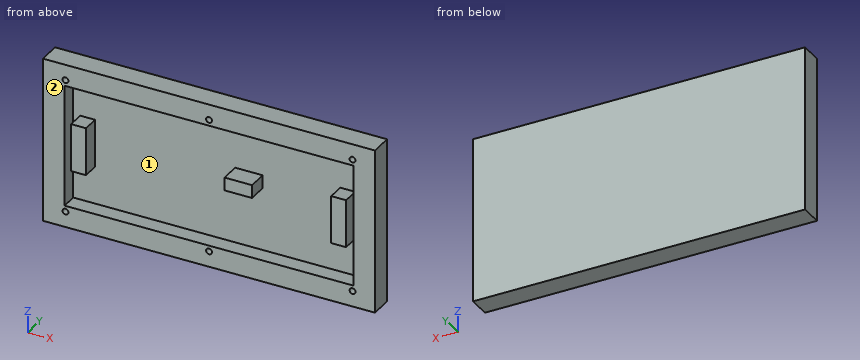
```python
from build123d import *

# Parameters (mm, degrees)
SKETCH1_W                = 192
SKETCH1_H                = 96
BOSS_EXTRUDE1_DEPTH      = 12.8
SKETCH2_W                = 167
SKETCH2_H                = 71
CUT_EXTRUDE1_DEPTH       = 9.2
M3_CLEARANCE_HOLE1_D     = 3.4
M3_CLEARANCE_HOLE1_DEPTH = 5
M3_CLEARANCE_HOLE1_TIP   = 1.021463052
SKETCH6_W                = 8.6
SKETCH6_H                = 27.8
BOSS_EXTRUDE2_DEPTH      = 9.6
SKETCH7_W                = 15.9
SKETCH7_H                = 7.6
BOSS_EXTRUDE3_DEPTH      = 11.2


with BuildPart() as part:
    # Sketch1 → Boss-Extrude1 (new body)
    with BuildSketch(Plane(origin=(0, 0, 0), x_dir=(1, 0, 0), z_dir=(0, 1, 0))):
        with Locations((96, 48)):
            Rectangle(SKETCH1_W, SKETCH1_H)
    extrude(amount=BOSS_EXTRUDE1_DEPTH)

    # Sketch2 → Cut-Extrude1 (cut)
    with BuildSketch(Plane.XZ):
        with Locations((96, -48)):
            Rectangle(SKETCH2_W, SKETCH2_H)
    extrude(amount=-CUT_EXTRUDE1_DEPTH, mode=Mode.SUBTRACT)

    # M3 Clearance Hole1
    with Locations(Plane(origin=(0, 0, 0), x_dir=(-1, 0, 0), z_dir=(0, -1, 0))):
        with Locations((-13, 9.1), (-96, 9.1), (-179, 9.1), (-179, 86.9), (-96, 86.9), (-13, 86.9)):
            Hole(M3_CLEARANCE_HOLE1_D / 2, depth=M3_CLEARANCE_HOLE1_DEPTH)
            with Locations((0, 0, -(M3_CLEARANCE_HOLE1_DEPTH + M3_CLEARANCE_HOLE1_TIP / 2))):  # 118° drill point
                Cone(0, M3_CLEARANCE_HOLE1_D / 2, M3_CLEARANCE_HOLE1_TIP, mode=Mode.SUBTRACT)

    # Sketch6 → Boss-Extrude2 (add)
    with BuildSketch(Plane.XZ.offset(-9.2)):
        with Locations((20.8, -47.8)):
            Rectangle(SKETCH6_W, SKETCH6_H)
        with Locations((171.2, -47.8)):
            Rectangle(SKETCH6_W, SKETCH6_H)
    extrude(amount=BOSS_EXTRUDE2_DEPTH)

    # Sketch7 → Boss-Extrude3 (add)
    with BuildSketch(Plane.XZ.offset(-9.2)):
        with Locations((114.05, -43.1)):
            Rectangle(SKETCH7_W, SKETCH7_H)
    extrude(amount=BOSS_EXTRUDE3_DEPTH)


solid = part.part
```
CAD build for the part. Positions are in the model's coordinates, mm. Face numbers are marked on the shaded views. Coordinates: 2 decimals unless noted, no trailing zeros. Write each loop counter-clockwise with the first axis right and the second up, starting at its lowest first coordinate (ties: lowest second). Pieces come first, ordered by that corner, then holes. Notation, with made-up numbers: (-5, 40) -> (20, 40) arc R15 ccw to (20, 59) -> close; hole circle Ø11 at (-11.75, 13.25). An arc over 180 degrees is marked (long way). Use CSV: the item, a comma, the result in double quotes. Start each with the question number.
Item 1: Band-saw the part on A-A, the plane y = 2.75. Give the number of separate pieces and of enclosed holes in the cut face, plus the area to 3 significant figures.
Item 2: Band-saw the part on B-B, the plane z = -25. Write the cut outline in (x, y).
Item 3: Band-saw the part on D-D, the plane z = -54.5. Write the cut outline in (x, y), plus the area to 3 significant figures.
Item 4: Wall check: probe 1 along Z at (x, y) = (13, 1.75); probe 2 along X at (y, z) = (4.5, -52); probe 3 along X at (y, z) = (1.5, -86.9). Give the ranges that are in metal, low to high.
Item 5: Drop flat-ended pins along their axis: P1, Ø2, axis at x = 96, z = -9.1, coming from the -Y side; P2, Ø2, axis at x = 57, z = -84, coming from the -Y side. Give the stop position or say it passes through.
Item 6: Band-saw the part on C-C, the plane x = 116. Write the cut outline in (y, z).
Item 7: Two-plate mould, pull along Z, no slides. Class the marked faces 1 and 2: +Z half, -Z half, draft (parallel to the pull), parting line (faces both ways), or undercut.
Response values:
1,separate pieces,"4"
1,enclosed holes,"7"
1,area,"7,120 mm2"
2,outline,"(0, 0) -> (12.5, 0) -> (12.5, 9.2) -> (179.5, 9.2) -> (179.5, 0) -> (192, 0) -> (192, 12.8) -> (0, 12.8) -> close"
3,outline,"(0, 0) -> (12.5, 0) -> (12.5, 9.2) -> (16.5, 9.2) -> (16.5, -0.4) -> (25.1, -0.4) -> (25.1, 9.2) -> (166.9, 9.2) -> (166.9, -0.4) -> (175.5, -0.4) -> (175.5, 9.2) -> (179.5, 9.2) -> (179.5, 0) -> (192, 0) -> (192, 12.8) -> (0, 12.8) -> close"
3,area,"1,090 mm2"
4,probe 1,"z = -96 to -88.6, -85.2 to -83.5, -12.5 to -10.8, -7.4 to 0"
4,probe 2,"x = 0 to 12.5, 16.5 to 25.1, 166.9 to 175.5, 179.5 to 192"
4,probe 3,"x = 0 to 11.3, 14.7 to 94.3, 97.7 to 177.3, 180.7 to 192"
5,P1,"stops at y = 5.42"
5,P2,"stops at y = 0"
6,outline,"(-2, -46.9) -> (9.2, -46.9) -> (9.2, -83.5) -> (0, -83.5) -> (0, -96) -> (12.8, -96) -> (12.8, 0) -> (0, 0) -> (0, -12.5) -> (9.2, -12.5) -> (9.2, -39.3) -> (-2, -39.3) -> close"
7,face 1,"undercut"
7,face 2,"draft"
